Geometry: final body of the model. Coordinates: model frame, mm. A direction names the side the tool comes from. Give positions to 0.01 mm unless a question says otherwise; leave off trailing zeros. Write each loop counter-clockwise with the first axis right and the second up, starting at its lowest first coordinate (ties: lowest second). Pieces come first, ordered by that corner, then holes.
Q1. Line query: L1, parallel to Z at x = 0, y = -4; L2, parallel to Y at x = -222, z = -179. Output: solid intervals per line, ascending.
Q2. Cut plane B-B on x = 116. Return the cut outline in (y, z).
Q3. Cut plane A-A on z = 75. Return the cut outline in (x, y), plus the area to 3 significant figures.
Q4. Cut plane D-D on z = 165.5. Return the cut outline in (x, y).
Q5. Pin query (flat end, axial travel): pin 1 (10 mm diameter, centred on x = -434, y = 10.5, fed in from +Z); pin 2 (12.5 mm diameter, centred on x = 0, z = 0, fed in from -Y); pin 3 (3 mm diameter, centred on x = -521, z = -286, fed in from +Y); pin 4 (10 mm diameter, centred on x = -243.5, y = 23.5, fed in from +Z). Return the tip coordinate at first contact, or that it passes through.
Q6. Cut plane C-C on y = 16. Return the cut outline in (x, z), plus the area to 3 significant figures.
Q7. Reachability of faces 4 (the face through (-261.626, 17.255, -450.547)), 5 (the face through (-172, -6.35, -133)), 6 (the face through (-520.986, -3.131, 3.819)) from +Z, -Z, +X, -X, +Y, -Y: full face, straight path, thin tool, end or side. Return the list, or none.
Q8. Draft query along Z for faces 1 (the face through (-263, 35, -456)), 2 (the face through (-268.864, 17.255, -457.901)), 3 (the face through (-530.986, -3.131, -3.892)). Return one class per face: pulls with the +Z half, pulls with the -Z half, needs draft (parallel to the pull), parting line crosses it, or undercut.
```python
from build123d import *

# Parameters (mm, degrees)
BOSS_EXTRUDE1_DEPTH    = 35
SKETCH4_W              = 1200
SKETCH4_H              = 806.4
BOSS_EXTRUDE2_DEPTH    = 6.35
CHAMFER1_SIZE          = 10
F_20_0MM_DOWEL_HOLE1_D = 21
CUT_EXTRUDE1_DEPTH     = 932.12242208


with BuildPart() as part:
    # Sketch3 → Boss-Extrude1 (new body)
    with BuildSketch(Plane(origin=(0, 0, 0), x_dir=(1, 0, 0), z_dir=(0, 1, 0))):
        with BuildLine():
            Line((0, 531), (0, 521))
            ThreePointArc((0, 521), (-260.5, 451.199235372), (-451.199235372, 260.5))
            Line((-451.199235372, 260.5), (-459.85948941, 265.5))
            ThreePointArc((-459.85948941, 265.5), (-265.5, 459.85948941), (0, 531))
        make_face()
    extrude(amount=BOSS_EXTRUDE1_DEPTH)

    # Sketch4 → Boss-Extrude2 (add)
    with BuildSketch(Plane(origin=(0, 0, 0), x_dir=(1, 0, 0), z_dir=(0, 1, 0))):
        with Locations((-164.07, 127.8)):
            Rectangle(SKETCH4_W, SKETCH4_H)
    extrude(amount=-BOSS_EXTRUDE2_DEPTH)

    # Chamfer1
    # the kernel refuses this chamfer: 10 mm, written as the material it takes off along each edge
    with BuildSketch(Plane(origin=(0, 0, -521), x_dir=(-0.999953038196086, 0, 0.009691305506332204), z_dir=(0, 1, 0))) as chamfer1_piece_1:
        with BuildLine():
            Line((10.098340338, 0), (-CHAMFER1_SIZE * 0.00969130550632, -CHAMFER1_SIZE * 0.999953038196))
            Line((-CHAMFER1_SIZE * 0.00969130550632, -CHAMFER1_SIZE * 0.999953038196), (0, 0))
            ThreePointArc((0, 0), (5.192000536, -0.024447522), (10.098340338, 0))
        make_face()
    extrude(amount=60.969219121, mode=Mode.SUBTRACT)

    # Ø20.0mm Dowel Hole1 (through all)
    with Locations(Plane(origin=(0, 0, 0), x_dir=(1, 0, 0), z_dir=(0, 1, 0))):
        with Locations((0, 0)):
            Hole(F_20_0MM_DOWEL_HOLE1_D / 2)

    # Sketch8 → Cut-Extrude1 (cut, through all)
    with BuildSketch(Plane(origin=(0, 0, 0), x_dir=(1, 0, 0), z_dir=(0, 1, 0))):
        with BuildLine():
            Line((-451.199235372, 260.5), (-459.85948941, 265.5))
            ThreePointArc((-459.85948941, 265.5), (-531, 0), (-459.85948941, -265.5))
            Line((-459.85948941, -265.5), (-451.199235372, -260.5))
            ThreePointArc((-451.199235372, -260.5), (-521, 0), (-451.199235372, 260.5))
        make_face()
    extrude(amount=-CUT_EXTRUDE1_DEPTH, mode=Mode.SUBTRACT)


solid = part.part
```
Data:
1. L1: z = -531 to -10.5, 10.5 to 275.4
1. L2: y = -6.35 to 0
2. outline: (-6.35, -531) - (0, -531) - (0, 275.4) - (-6.35, 275.4) - close
3. outline: (-764.07, -6.35) - (-525.68, -6.35) - (-525.68, 0) - (-764.07, 0) - close; (-515.57, -6.35) - (435.93, -6.35) - (435.93, 0) - (-515.57, 0) - close
3. area: 7,560 mm2
4. outline: (-764.07, -6.35) - (-504.55, -6.35) - (-504.55, 0) - (-764.07, 0) - close; (-494.01, -6.35) - (435.93, -6.35) - (435.93, 0) - (-494.01, 0) - close
5. pin 1: stops at z = -280.57
5. pin 2: passes through
5. pin 3: stops at y = 0
5. pin 4: stops at z = -457.92
6. outline: (-459.86, -265.5) arc R531 ccw to (0, -531) - (-10.1, -520.9) arc R521 cw to (-451.2, -260.5) - close
6. area: 5,460 mm2
7. face 4: +Z, +X, +Y
7. face 5: +Z, -Z, +X, -X, -Y
7. face 6: +Y, -Y
8. face 1: needs draft
8. face 2: pulls with the -Z half
8. face 3: undercut
